Check sheet for the modelled part. Datum: model origin and axes. Units: mm. Face numbers are marked on the shaded views. Round coordinates to 2 decimals unless told otherwise and drop trailing zeros. Loops run counter-clockwise (first coordinate to the right, second up) from the corner with the lowest first, then second, coordinate; pieces in that order, holes last. Notation, with made-up numbers: (85.25, 87.5) -> (96.25, 87.5) arc R32 cw to (96.25, 114.5) -> close; hole circle Ø6 at (52, -33.75). An arc over 180 degrees is marked (long way). Return JSON: item names as keys, results as strings.
from build123d import *

# Parameters (mm, degrees)
CUT_EXTRUDE8_REACH      = 118.862
CUT_EXTRUDE8_END_RADIUS = 3
SKETCH2_R               = 2.5
SKETCH9_R               = 5
CUT_EXTRUDE9_DEPTH      = 5
CHAMFER1_SIZE           = 2.5


with BuildPart() as part:
    # Sketch1 → Revolve1 (revolve)
    with BuildSketch(Plane.XY, mode=Mode.PRIVATE) as revolve1_sk:
        with BuildLine():
            Line((-28.837765837, -3), (-15.779224455, -3))
            Line((-15.779224455, -3), (-15.779224455, 0))
            Line((-15.779224455, 0), (-8.279224455, 0))
            Line((-8.279224455, 0), (-8.279224455, -46.741129743))
            Line((-8.279224455, -46.741129743), (-39.621237636, -46.741129743))
            ThreePointArc((-39.621237636, -46.741129743), (-41.576881329, -44.736133736), (-44.279224455, -44))
            Line((-44.279224455, -44), (-44.279224455, -42))
            Line((-44.279224455, -42), (-52.279224455, -42))
            Line((-52.279224455, -42), (-52.279224455, -30))
            Line((-52.279224455, -30), (-52.279224455, -24.707456133))
            Line((-52.279224455, -24.707456133), (-50.558495146, -22.25))
            Line((-50.558495146, -22.25), (-50.558495146, -5.457456133))
            Line((-50.558495146, -5.457456133), (-48.837765837, -3))
            Line((-48.837765837, -3), (-28.837765837, -3))
        make_face()
    revolve(revolve1_sk.sketch.rotate(Axis((-82.123840877, 0, 0), (1, 0, 0)), 270), axis=Axis((-82.123840877, 0, 0), (1, 0, 0)))

    # Cut-Extrude8: up to this cylinder (the profile starts outside it)
    cut_extrude8_end = Plane(origin=(-18.279224, 0, 0), z_dir=(-1, 0, 0)) * Cylinder(CUT_EXTRUDE8_END_RADIUS, 244.724, mode=Mode.PRIVATE)
    # Sketch2 → Cut-Extrude8 (cut, up to the surface)
    with BuildSketch(Plane.XY.offset(46.741129743), mode=Mode.PRIVATE) as cut_extrude8_sk1:
        with Locations((-18.279224455, 0)):
            Circle(SKETCH2_R)
    cut_extrude8_tool1 = extrude(cut_extrude8_sk1.sketch, amount=-CUT_EXTRUDE8_REACH, mode=Mode.PRIVATE) - cut_extrude8_end
    add(cut_extrude8_tool1.solids().sort_by_distance((-18.279224, 0, 46.74113))[0], mode=Mode.SUBTRACT)

    # Sketch9 → Cut-Extrude9 (cut)
    with BuildSketch(Plane.XY.offset(46.741129743)):
        with Locations((-18.279224455, 0)):
            Circle(SKETCH9_R)
    extrude(amount=-CUT_EXTRUDE9_DEPTH, mode=Mode.SUBTRACT)

    # Chamfer1
    chamfer1_edges = [part.edges().sort_by_distance(p)[0] for p in [
        (-20.779224455, 0, 41.741129743),
    ]]
    chamfer(chamfer1_edges, length=CHAMFER1_SIZE - 0.0001)  # a hair under: the kernel refuses the full size


solid = part.part
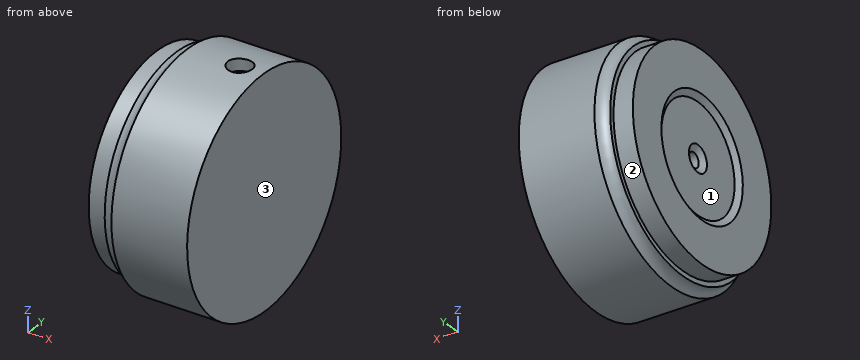
Q1. Material ranges on line 1 (Y direction, x = -38.5, z = 0); line 2 (Y direction, x = -40, z = 0); line 3 (Z direction, x = -24.5, y = -20.5), recorded low to high.
Results list:
{"line 1": "-46.74 to -3, 3 to 46.74", "line 2": "-46.15 to -3, 3 to 46.15", "line 3": "-42.01 to 42.01"}
Q2. Section check B-B (x = -32). Record the boundary of the cut face in (y, z), then the cut area to 3 significant figures.
Results list:
{"outline": "circle Ø93.48 at (0, 0); hole circle Ø6 at (0, 0)", "area": "6,840 mm^2"}
Q3. Go/stop test with flat-tipped pins: pin 1 (10 mm diameter, centred on x = -44, y = 9, fed in from +Z); pin 2 (4 mm diameter, centred on y = 33, z = 34.5, fed in from -X); pin 3 (12 mm diameter, centred on x = -43, z = 12.5, fed in from +Y); pin 4 (10 mm diameter, centred on x = -24, y = 5, fed in from -Z). Record where each tip stops, or that it passes through.
Results list:
{"pin 1": "z = 46.27", "pin 2": "x = -40.34", "pin 3": "y = 46.13", "pin 4": "z = -46.74"}
Q4. Section check C-C (x = -42.5). Record the boundary of the cut face in (y, z).
Results list:
{"outline": "circle Ø88.61 at (0, 0); hole circle Ø6 at (0, 0)"}
Q5. Draft check along Z on the marked faces 1, 2 and 3. Enter one of: released by +Z, released by -Z, zero draft, split by the parting line, or undercut.
Results list:
{"face 1": "undercut", "face 2": "split by the parting line", "face 3": "zero draft"}
Q6. Section check A-A (z = 0). Record the boundary of the cut face in (x, y), then the cut area to 3 significant figures.
Results list:
{"outline": "(-52.28, -42) -> (-44.28, -42) -> (-44.28, -44) arc R5.33 cw to (-39.62, -46.74) -> (-8.28, -46.74) -> (-8.28, 46.74) -> (-39.62, 46.74) arc R5.33 cw to (-44.28, 44) -> (-44.28, 42) -> (-52.28, 42) -> (-52.28, 24.71) -> (-50.56, 22.25) -> (-50.56, 5.46) -> (-48.84, 3) -> (-15.78, 3) -> (-15.78, -3) -> (-48.84, -3) -> (-50.56, -5.46) -> (-50.56, -22.25) -> (-52.28, -24.71) -> close", "area": "3,730 mm^2"}
